Autodesk Inventor part; units mm, degrees
ref_plane "YZ Plane" through (0, 0, 0) normal (1, 0, 0) x (0, 1, 0)
ref_plane "XZ Plane" through (0, 0, 0) normal (0, 1, 0) x (-1, 0, 0)
ref_plane "XY Plane" through (0, 0, 0) normal (0, 0, 1) x (1, 0, 0)
sketch "Sketch1" plane through (0, 0, 0) normal (0, 0, 1) x (1, 0, 0)
  line L0 (-28.575, -28.575) -> (28.575, -28.575)
  line L1 (28.575, -28.575) -> (28.575, 28.575)
  line L2 (28.575, 28.575) -> (-28.575, 28.575)
  line L3 (-28.575, 28.575) -> (-28.575, -28.575)
  line L4 (-28.575, -28.575) -> (28.575, 28.575) construction
  line L5 (28.575, -28.575) -> (-28.575, 28.575) construction
  line L6 (-28.575, 0) -> (28.575, 0) construction
  line L7 (0, 28.575) -> (0, -28.575) construction
  circle A0 centre (-24.765, 24.765) radius 1.3
  circle A1 centre (24.765, 24.765) radius 1.3
  circle A2 centre (-24.765, -24.765) radius 1.3
  circle A3 centre (24.765, -24.765) radius 1.3
  point P0 (0, 0)
  dimension "d2" = 57.15
  dimension "d4" = 57.15
  dimension "d26" = 2.6
  dimension "d27" = 3.81
extrude "Extrusion1" add sketch "Sketch1" along normal blind 1.64
sketch "Sketch4" plane through (0, 0, 0) normal (0, 0, -1) x (-1, 0, 0)
  line L0 (-28.575, -28.575) -> (28.575, -28.575)
  line L1 (-28.575, 28.575) -> (-28.575, -28.575)
  line L2 (-26.575, 18.5) -> (-20.275, 18.5)
  line L3 (-20.275, 18.5) -> (-20.275, -18.5)
  line L4 (-20.275, -18.5) -> (-26.575, -18.5)
  line L5 (-26.575, -18.5) -> (-26.575, 18.5)
  line L6 (-20.275, 18.5) -> (-26.575, -18.5) construction
  line L7 (-26.575, 18.5) -> (-20.275, -18.5) construction
  line L8 (0, 0) -> (-28.575, 0) construction
  line L9 (0, -28.575) -> (0, 0) construction
  line L10 (26.575, 18.5) -> (20.275, 18.5)
  line L11 (20.275, 18.5) -> (20.275, -18.5)
  line L12 (20.275, -18.5) -> (26.575, -18.5)
  line L13 (26.575, -18.5) -> (26.575, 18.5)
  line L14 (28.575, -28.575) -> (-28.575, -28.575)
  line L15 (28.575, 28.575) -> (28.575, -28.575)
  line L16 (-28.575, 28.575) -> (28.575, 28.575)
  line L17 (-28.575, -28.575) -> (-28.575, 28.575)
  point P0 (-23.425, 0)
  dimension "d21" = 37
  dimension "d22" = 6.3
  dimension "d23" = 2
extrude "Extrusion4" add sketch "Sketch4" along normal blind 5 contours L2 L3 L4 L5 | L13 L12 L11 L10
properties part number "SFE-ProcessingBoard01" material "PCB(1)"
CAD build for the part. Positions are in the model's coordinates, mm. A direction names the side the tool comes from. Give positions to 0.01 mm unless a question says otherwise; leave off trailing zeros. Write each loop counter-clockwise with the first axis right and the second up, starting at its lowest first coordinate (ties: lowest second). Pieces come first, ordered by that corner, then holes. Notation, with made-up numbers: M -20.5,34.25 L 11.5,34.25 A6 cw 11.5,40.25 Z; hole C -28.75,-4.5 d3. An arc over 180 degrees is marked long. Return JSON: item names as keys, results as strings. Group by question number.
(1) Band-saw the part on A-A (z = -4). Give the cut face in (x, y) (3 decimals), and give its area (3 significant figures).
(2) Drill centre lines: L1, parallel to X at y = 2.5, z = -3.25 (3 decimals); L2, parallel to Z at x = 13, y = 22; L3, parallel to Y at x = -22, z = -0.75. Where is each one in solid material? Low to high. Write a range as [from, to].
(3) 3-axis set-ups, long thin cutter, end or side, ignore diameter. For faces 4 (the face through (26.575, 0, -2)), 5 (the face through (-23, 18.5, -2)), 6 (the face through (-20.275, 0, -2)): which of +Z, -Z, +X, -X, +Y, -Y reach the whole face in a straight line?
(4) Band-saw the part on D-D (y = -21). Give the cut face in (x, z) (3 decimals).
(5) Band-saw the part on C-C (y = 1). Give the cut face in (x, z) (3 decimals).
(6) Mould opens along Y. For faces 1 (the face through (25.464, 23.669, 0.809)), 2 (the face through (-23, 0, -5)), 3 (the face through (23, 18.5, -2)) say: pulls with the +Y half, pulls with the -Y half, needs draft (parallel to the pull), parting line crosses it, or undercut.
(7) Band-saw the part on B-B (x = -22.5). Give the cut face in (y, z) (3 decimals).
(8) Flat gauge pins, fed straight in: pin 1 Ø1.5 at (y, z) = (-2, -3) entering from +X (3 decimals); pin 2 Ø3 at (x, y) = (24.765, 24.765) entering from -Z; pin 3 Ø2.5 at (x, z) = (-23.5, -1.5) entering from -Y. Where does each tip first touch, or does it go through?
Entries:
{
 "1": {"outline": "M -26.575,-18.5 L -20.275,-18.5 L -20.275,18.5 L -26.575,18.5 Z; M 20.275,-18.5 L 26.575,-18.5 L 26.575,18.5 L 20.275,18.5 Z", "area": "466 mm^2"},
 "2": {"L1": "x = [-26.575, -20.275], [20.275, 26.575]", "L2": "z = [0, 1.64]", "L3": "y = [-18.5, 18.5]"},
 "3": {"face 4": "-Z, +X, +Y, -Y", "face 5": "-Z, +X, -X, +Y", "face 6": "-Z, +Y, -Y"},
 "4": {"outline": "M -28.575,0 L 28.575,0 L 28.575,1.64 L -28.575,1.64 Z"},
 "5": {"outline": "M -28.575,0 L -26.575,0 L -26.575,-5 L -20.275,-5 L -20.275,0 L 20.275,0 L 20.275,-5 L 26.575,-5 L 26.575,0 L 28.575,0 L 28.575,1.64 L -28.575,1.64 Z"},
 "6": {"face 1": "undercut", "face 2": "needs draft", "face 3": "pulls with the +Y half"},
 "7": {"outline": "M -28.575,0 L -18.5,0 L -18.5,-5 L 18.5,-5 L 18.5,0 L 28.575,0 L 28.575,1.64 L -28.575,1.64 Z"},
 "8": {"pin 1": "stops at x = 26.575", "pin 2": "stops at z = 0", "pin 3": "stops at y = -18.5"}
}
